Work out the finished part from the listing and answer in its coordinate system (mm). Face numbers are marked on the shaded views. A direction names the side the tool comes from. Give positions to 0.01 mm unless a question says otherwise; leave off trailing zeros. Write each loop counter-clockwise with the first axis right and the second up, starting at its lowest first coordinate (ties: lowest second). Pieces come first, ordered by that corner, then holes. Notation, with made-up numbers: (26, -6) -> (70, -6) arc R29 cw to (70, 25) -> close; hole circle Ø6 at (76, 2). An arc over 180 degrees is marked (long way). Use a Markdown table: item, result. Add a question column.
Q1. Each of these flat-tipped pins is pushed along its axis until it touches: pin 1 Ø2.5 at (x, z) = (49, -18.5) entering from +Y; pin 2 Ø12 at (x, z) = (29, -30) entering from +Y; pin 3 Ø2 at (x, y) = (32, 5.5) entering from +Z. Where does it stop, or does it pass through?
Q2. Section B-B, the plane z = -20.05 is taken. Give the vertices of the cut face in (x, y).
Q3. Section A-A, the plane y = 5.25 is taken. Give the vertices of the cut face in (x, z), plus the area to 3 significant figures.
Q4. Section C-C, the plane x = 47.75 is taken. Give the vertices of the cut face in (y, z).
Q5. For the marked faces 1 and 2, determine the directions among +Z, -Z, +X, -X, +Y, -Y from which every point of the face is accessible in a straight line to the end or side of a thin tool.
Q6. Section D-D, the plane y = 8.75 is taken. Give the vertices of the cut face in (x, z), plus the area to 3 significant figures.
Q7. Consider line 1 (X direction, y = 4, z = -20.05); line 2 (Z direction, x = 47.75, y = 3.8); line 3 (Z direction, x = 23, y = 7.5). Determine where each line is inside the solid, lowest interval first.
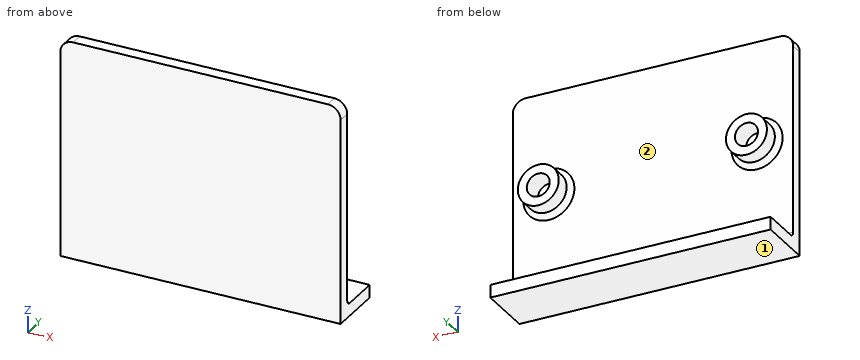
Autodesk Inventor part; units mm, degrees
ref_plane "YZ Plane" through (0, 0, 0) normal (1, 0, 0) x (0, 1, 0)
ref_plane "XZ Plane" through (0, 0, 0) normal (0, 1, 0) x (-1, 0, 0)
ref_plane "XY Plane" through (0, 0, 0) normal (0, 0, 1) x (1, 0, 0)
sketch "Sketch1" plane through (0, 0, 0) normal (0, 1, 0) x (-1, 0, 0)
  line L0 (0, 0) -> (-54.8, 0)
  line L1 (-54.8, 0) -> (-54.8, -42.6)
  line L2 (-54.8, -42.6) -> (0, -42.6)
  line L3 (0, -42.6) -> (0, 0)
  dimension "d0" = 54.8
  dimension "d1" = 42.6
extrude "Extrusion1" add sketch "Sketch1" along normal blind 2.5
sketch "Sketch2" plane through (0, 2.5, 0) normal (0, 1, 0) x (1, 0, 0)
  line L0 (54.8, 0) -> (54.8, 42.6)
  line L1 (54.8, 42.6) -> (0, 42.6)
  line L2 (0, 42.6) -> (0, 0)
  line L3 (0, 0) -> (54.8, 0)
  line L4 (0, 42.6) -> (54.8, 42.6)
  line L5 (54.8, 42.6) -> (54.8, 40.1)
  line L6 (54.8, 40.1) -> (0, 40.1)
  line L7 (0, 40.1) -> (0, 42.6)
  dimension "d4" = 2.5
extrude "Extrusion2" add sketch "Sketch2" along normal blind 8.5 contours L6 L2 L1 L0
sketch "Sketch3" plane through (0, 2.5, 0) normal (0, 1, 0) x (1, 0, 0)
  line L0 (54.8, 40.1) -> (0, 40.1)
  line L1 (0, 40.1) -> (0, 0)
  line L2 (0, 0) -> (54.8, 0)
  line L3 (54.8, 0) -> (54.8, 40.1)
  circle A0 centre (7.05, 20.05) radius 4
  circle A1 centre (47.75, 20.05) radius 4
  dimension "d7" = 8
  dimension "d8" = 8
  dimension "d9" = 7.05
  dimension "d10" = 7.05
  dimension "d11" = 20.05
  dimension "d12" = 20.05
extrude "Extrusion3" cut sketch "Sketch3" against normal blind 0.5 contours A0 | A1
sketch "Sketch4" plane through (7.05, 2, -20.05) normal (0, 1, 0) x (1, 0, 0)
  circle A0 centre (0, 0) radius 4
  circle A1 centre (0, 0) radius 4
  circle A2 centre (40.7, 0) radius 4
  circle A3 centre (40.7, 0) radius 4
  point P0 (-7.05, -20.05)
  dimension "d15" = 8
  dimension "d16" = 8
extrude "Extrusion4" add sketch "Sketch4" along normal blind 4.5
sketch "Sketch5" plane through (7.05, 6.5, -20.05) normal (0, 1, 0) x (1, 0, 0)
  circle A0 centre (0, 0) radius 4
  circle A1 centre (0, 0) radius 2.25
  circle A2 centre (40.7, 0) radius 4
  circle A3 centre (40.7, 0) radius 2.25
  point P0 (-7.05, -20.05)
  dimension "d19" = 4.5
  dimension "d20" = 4.5
extrude "Extrusion5" cut sketch "Sketch5" against normal blind 4.2 contours A1 | A3
chamfer "Chamfer1" distance 1 angle 45 2 edges at (3.05, 2.5, -20.05) (43.75, 2.5, -20.05)
fillet "Fillet1" radius 2.5 2 edges at (0, 1.25, 0) (54.8, 1.25, 0)
fillet "Fillet2" radius 1 1 edges at (27.4, 2.5, -40.1)
properties part number "small_backplate"
Result set:
| question | item | result |
|---|---|---|
| 1 | pin 1 | stops at y = 6.5 |
| 1 | pin 2 | stops at y = 2.5 |
| 1 | pin 3 | stops at z = -40.1 |
| 2 | outline | (0, 0) -> (54.8, 0) -> (54.8, 2.5) -> (52.75, 2.5) -> (51.75, 3.5) -> (51.75, 6.5) -> (50, 6.5) -> (50, 2.3) -> (45.5, 2.3) -> (45.5, 6.5) -> (43.75, 6.5) -> (43.75, 3.5) -> (42.75, 2.5) -> (12.05, 2.5) -> (11.05, 3.5) -> (11.05, 6.5) -> (9.3, 6.5) -> (9.3, 2.3) -> (4.8, 2.3) -> (4.8, 6.5) -> (3.05, 6.5) -> (3.05, 3.5) -> (2.05, 2.5) -> (0, 2.5) -> close |
| 3 | outline | (0, -42.6) -> (54.8, -42.6) -> (54.8, -40.1) -> (0, -40.1) -> close; circle Ø8 at (7.05, -20.05); circle Ø8 at (47.75, -20.05); hole circle Ø4.5 at (7.05, -20.05); hole circle Ø4.5 at (47.75, -20.05) |
| 3 | area | 206 mm2 |
| 4 | outline | (0, -42.6) -> (11, -42.6) -> (11, -40.1) -> (3.5, -40.1) arc R1 cw to (2.5, -39.1) -> (2.5, -25.05) -> (3.5, -24.05) -> (6.5, -24.05) -> (6.5, -22.3) -> (2.3, -22.3) -> (2.3, -17.8) -> (6.5, -17.8) -> (6.5, -16.05) -> (3.5, -16.05) -> (2.5, -15.05) -> (2.5, 0) -> (0, 0) -> close |
| 5 | face 1 | -Z, +X, -X, +Y, -Y |
| 5 | face 2 | +Y |
| 6 | outline | (0, -42.6) -> (54.8, -42.6) -> (54.8, -40.1) -> (0, -40.1) -> close |
| 6 | area | 137 mm2 |
| 7 | line 1 | x = 3.05 to 4.8, 9.3 to 11.05, 43.75 to 45.5, 50 to 51.75 |
| 7 | line 2 | z = -42.6 to -40.1, -24.05 to -22.3, -17.8 to -16.05 |
| 7 | line 3 | z = -42.6 to -40.1 |
